Source: CAD feature listing. Evaluate the final solid. Frame: model axes, mm. Face numbers are marked on the shaded views. A direction names the side the tool comes from. Round coordinates to 2 decimals unless told otherwise and drop trailing zeros. Order: outer loops, then holes, each group sorted by start corner. A loop starts at its lowest first (then second) coordinate and runs counter-clockwise, first axis right, second up. Notation, with made-up numbers: (48, 56) - (82, 56) arc R26 cw to (82, 84) - close; hole circle Ø4 at (59.5, 39.5). An arc over 180 degrees is marked (long way). Put each result on its own line as item: value. Start each with the question number.
1) Access query for the marked faces 1 and 2. Directions: +Z, -Z, +X, -X, +Y, -Y. A direction counts if a zero-diameter tool reaches every point of the face in a straight line with its end or side. Return the directions, or none.
2) Section C-C on x = -20. Output: boundary loops of the cut face in (y, z).
3) Contact query for flat-ended pins moving along their axis: P1, Ø1.5, axis at y = 13, z = 7, coming from the +X side; P2, Ø3, axis at y = 20.5, z = -14, coming from the -X side; P3, Ø4, axis at x = 21.05, z = 15.875, coming from the +Y side. Output: stop coordinate, or through.
4) Section A-A on x = -10.7. Output: boundary loops of the cut face in (y, z), then the cut area to 3 significant figures.
5) Section D-D on y = 6. Output: boundary loops of the cut face in (x, z).
6) Line query: probe 1 along Y at (x, z) = (10, -12.5); probe 2 along X at (y, z) = (13.5, 12); probe 3 along Y at (x, z) = (-23, 9). Output: solid intervals per line, ascending. Write a range as [from, to].
```python
from build123d import *

# Parameters (mm, degrees)
SKETCH1_W               = 50.8
SKETCH1_H               = 38.1
BOSS_EXTRUDE1_DEPTH     = 2
SKETCH2_W               = 2
SKETCH2_H               = 38.1
BOSS_EXTRUDE2_DEPTH     = 38.1
CUT_EXTRUDE2_DEPTH      = 38.1
SKETCH4_R               = 1.5875
CUT_EXTRUDE3_DEPTH      = 2
LPATTERN1_COUNT         = 7
LPATTERN1_PITCH         = 6.35
MIRROR1_COPY_1_SKETCH_R = 1.5875
MIRROR1_COPY_1_DEPTH    = 2
MIRROR1_COPY_2_SKETCH_R = 1.5875
MIRROR1_COPY_2_DEPTH    = 2
MIRROR1_COPY_3_SKETCH_R = 1.5875
MIRROR1_COPY_3_DEPTH    = 2
MIRROR1_COPY_4_SKETCH_R = 1.5875
MIRROR1_COPY_4_DEPTH    = 2
MIRROR1_COPY_5_SKETCH_R = 1.5875
MIRROR1_COPY_5_DEPTH    = 2
MIRROR1_COPY_6_SKETCH_R = 1.5875
MIRROR1_COPY_6_DEPTH    = 2
FILLET1_R               = 3.175
FILLET2_R               = 1.5875
FILLET3_R               = 3.175
SKETCH5_R               = 1.5875
CUT_EXTRUDE4_DEPTH      = 68.46519473


with BuildPart() as part:
    # Sketch1 → Boss-Extrude1 (new body)
    with BuildSketch(Plane(origin=(0, 0, 0), x_dir=(1, 0, 0), z_dir=(0, 1, 0))):
        Rectangle(SKETCH1_W, SKETCH1_H)
    extrude(amount=BOSS_EXTRUDE1_DEPTH)

    # Sketch2 → Boss-Extrude2 (add)
    with BuildSketch(Plane(origin=(0, 2, 0), x_dir=(1, 0, 0), z_dir=(0, 1, 0))):
        with Locations((-24.4, 0)):
            Rectangle(SKETCH2_W, SKETCH2_H)
    extrude(amount=BOSS_EXTRUDE2_DEPTH)

    # Sketch3 → Cut-Extrude2 (cut)
    with BuildSketch(Plane.ZY.offset(25.4)):
        with BuildLine():
            Line((19.05, 40.1), (0, 40.1))
            ThreePointArc((0, 40.1), (13.138759324, 34.85352032), (19.05, 22.000124688))
            Line((19.05, 22.000124688), (19.05, 40.1))
        make_face()
        with BuildLine():
            Line((-19.05, 40.1), (-19.05, 22.000124688))
            ThreePointArc((-19.05, 22.000124688), (-13.138759324, 34.85352032), (0, 40.1))
            Line((0, 40.1), (-19.05, 40.1))
        make_face()
    extrude(amount=-CUT_EXTRUDE2_DEPTH, mode=Mode.SUBTRACT)

    # Sketch4 → Cut-Extrude3 (cut)
    with BuildSketch(Plane(origin=(0, 2, 0), x_dir=(1, 0, 0), z_dir=(0, 1, 0))):
        with Locations(Location((-17.05, 15.875, 0), (0, 0, 270))):
            Circle(SKETCH4_R)
    cut_extrude3 = extrude(amount=-CUT_EXTRUDE3_DEPTH, mode=Mode.SUBTRACT)

    # LPattern1: Cut-Extrude3 ×7
    with Locations(*[(i * LPATTERN1_PITCH, 0, 0) for i in range(1, LPATTERN1_COUNT)]):
        add(cut_extrude3, mode=Mode.SUBTRACT)

    # Mirror1: Cut-Extrude3 across plane
    add(cut_extrude3.mirror(Plane.XY), mode=Mode.SUBTRACT)

    # Mirror1 copy 1 sketch → Mirror1 copy 1 (cut)
    with BuildSketch(Plane(origin=(6.35, 2, 0), x_dir=(1, 0, 0), z_dir=(0, 1, 0))):
        with Locations((-17.05, -15.875)):
            Circle(MIRROR1_COPY_1_SKETCH_R)
    extrude(amount=-MIRROR1_COPY_1_DEPTH, mode=Mode.SUBTRACT)

    # Mirror1 copy 2 sketch → Mirror1 copy 2 (cut)
    with BuildSketch(Plane(origin=(12.7, 2, 0), x_dir=(1, 0, 0), z_dir=(0, 1, 0))):
        with Locations((-17.05, -15.875)):
            Circle(MIRROR1_COPY_2_SKETCH_R)
    extrude(amount=-MIRROR1_COPY_2_DEPTH, mode=Mode.SUBTRACT)

    # Mirror1 copy 3 sketch → Mirror1 copy 3 (cut)
    with BuildSketch(Plane(origin=(19.05, 2, 0), x_dir=(1, 0, 0), z_dir=(0, 1, 0))):
        with Locations((-17.05, -15.875)):
            Circle(MIRROR1_COPY_3_SKETCH_R)
    extrude(amount=-MIRROR1_COPY_3_DEPTH, mode=Mode.SUBTRACT)

    # Mirror1 copy 4 sketch → Mirror1 copy 4 (cut)
    with BuildSketch(Plane(origin=(25.4, 2, 0), x_dir=(1, 0, 0), z_dir=(0, 1, 0))):
        with Locations((-17.05, -15.875)):
            Circle(MIRROR1_COPY_4_SKETCH_R)
    extrude(amount=-MIRROR1_COPY_4_DEPTH, mode=Mode.SUBTRACT)

    # Mirror1 copy 5 sketch → Mirror1 copy 5 (cut)
    with BuildSketch(Plane(origin=(31.75, 2, 0), x_dir=(1, 0, 0), z_dir=(0, 1, 0))):
        with Locations((-17.05, -15.875)):
            Circle(MIRROR1_COPY_5_SKETCH_R)
    extrude(amount=-MIRROR1_COPY_5_DEPTH, mode=Mode.SUBTRACT)

    # Mirror1 copy 6 sketch → Mirror1 copy 6 (cut)
    with BuildSketch(Plane(origin=(38.1, 2, 0), x_dir=(1, 0, 0), z_dir=(0, 1, 0))):
        with Locations((-17.05, -15.875)):
            Circle(MIRROR1_COPY_6_SKETCH_R)
    extrude(amount=-MIRROR1_COPY_6_DEPTH, mode=Mode.SUBTRACT)

    # Fillet1
    fillet1_edges = [part.edges().sort_by_distance(p)[0] for p in [
        (25.4, 1, 19.05),
        (25.4, 1, -19.05),
    ]]
    fillet(fillet1_edges, radius=FILLET1_R)

    # Fillet2
    fillet2_edges = [part.edges().sort_by_distance(p)[0] for p in [
        (-23.4, 2, 0),
    ]]
    fillet(fillet2_edges, radius=FILLET2_R)

    # Fillet3
    fillet3_edges = [part.edges().sort_by_distance(p)[0] for p in [
        (-25.4, 0, 0),
    ]]
    fillet(fillet3_edges, radius=FILLET3_R)

    # Sketch5 → Cut-Extrude4 (cut, through all)
    with BuildSketch(Plane.ZY.offset(25.4)):
        with Locations((14.2875, 21.6375)):
            Circle(SKETCH5_R)
        with Locations((7.14375, 9.264162043)):
            Circle(SKETCH5_R)
        with Locations((-7.14375, 9.264162043)):
            Circle(SKETCH5_R)
        with Locations((-14.2875, 21.6375)):
            Circle(SKETCH5_R)
        with Locations((-7.14375, 34.010837957)):
            Circle(SKETCH5_R)
        with Locations((7.14375, 34.010837957)):
            Circle(SKETCH5_R)
        with BuildLine():
            Line((-6.35, 27.9875), (-6.35, 15.2875))
            ThreePointArc((-6.35, 15.2875), (0, 8.9375), (6.35, 15.2875))
            Line((6.35, 15.2875), (6.35, 27.9875))
            ThreePointArc((6.35, 27.9875), (0, 34.3375), (-6.35, 27.9875))
        make_face()
    extrude(amount=-CUT_EXTRUDE4_DEPTH, mode=Mode.SUBTRACT)


solid = part.part
```
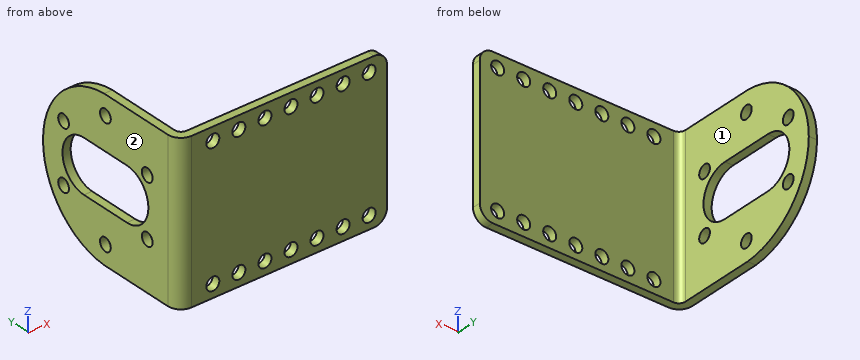
Answer sheet:
1. face 1: +Z, -Z, +X, +Y
1. face 2: +Z, -Z, -X, +Y, -Y
2. outline: (0, -19.05) - (2, -19.05) - (2, 19.05) - (0, 19.05) - close
3. P1: x = -23.4
3. P2: x = -25.4
3. P3: y = 2
4. outline: (0, -19.05) - (2, -19.05) - (2, -17.46) - (0, -17.46) - close; (0, -14.29) - (2, -14.29) - (2, 14.29) - (0, 14.29) - close; (0, 17.46) - (2, 17.46) - (2, 19.05) - (0, 19.05) - close
4. area: 63.5 mm^2
5. outline: (-25.4, -19.05) - (-23.4, -19.05) - (-23.4, 19.05) - (-25.4, 19.05) - close
6. probe 1: [0, 2]
6. probe 2: [-25.4, -23.4]
6. probe 3: [0.1, 2.53]
